```python
from build123d import *

# Parameters (mm, degrees)
SKETCH1_W                        = 40.9
SKETCH1_H                        = 40.9
BOSS_EXTRUDE1_DEPTH              = 40
CUT_EXTRUDE1_START               = -30.475
SKETCH3_W                        = 28.2
SKETCH3_H                        = 28.2
CUT_EXTRUDE1_DEPTH               = 30.475
FILLET1_R                        = 9.525
CIRPATTERN1_COUNT                = 2
CIRPATTERN1_ANGLE                = 90
SKETCH6_W                        = 2.5527
SKETCH6_H                        = 9.525
F_1_4_20_TAPPED_HOLE1_AT_2_COUNT = 2
F_1_4_20_TAPPED_HOLE1_AT_2_PITCH = 19.05
F_1_4_20_TAPPED_HOLE1_AT_3_COUNT = 2
F_1_4_20_TAPPED_HOLE1_AT_3_PITCH = 26.940768363
F_1_4_20_TAPPED_HOLE1_AT_4_COUNT = 2
F_1_4_20_TAPPED_HOLE1_AT_4_PITCH = 19.05


with BuildPart() as part:
    # Sketch1 → Boss-Extrude1 (new body)
    with BuildSketch(Plane(origin=(0, 0, 0), x_dir=(1, 0, 0), z_dir=(0, 1, 0))):
        Rectangle(SKETCH1_W, SKETCH1_H)
    extrude(amount=BOSS_EXTRUDE1_DEPTH)

    # Sketch3 → Cut-Extrude1 (cut)
    with BuildSketch(Plane(origin=(0, 40, 0), x_dir=(1, 0, 0), z_dir=(0, 1, 0)).offset(CUT_EXTRUDE1_START)):
        Rectangle(SKETCH3_W, SKETCH3_H)
    extrude(amount=CUT_EXTRUDE1_DEPTH, mode=Mode.SUBTRACT)

    # Fillet1
    fillet1_edges = [part.edges().sort_by_distance(p)[0] for p in [
        (14.1, 24.7625, 14.1),
        (14.1, 24.7625, -14.1),
        (-14.1, 24.7625, -14.1),
        (-14.1, 24.7625, 14.1),
    ]]
    fillet(fillet1_edges, radius=FILLET1_R)

    # Sketch4 → 5/16-18 Tapped Hole1 (revolve, cut)
    with BuildSketch(Plane(origin=(0, 25, 20.45), x_dir=(0, -1, 0), z_dir=(1, 0, 0))):
        Polygon((0, 0), (0, 24.884648974), (3.2639, 22.9235), (3.2639, 0), align=None)
    f_5_16_18_tapped_hole1 = revolve(axis=Axis((0, 25, 26.8), (0, 0, -1)), mode=Mode.SUBTRACT)

    # CirPattern1: 5/16-18 Tapped Hole1 ×2 about axis
    cirpattern1_axis = Axis((0, -2, 0), (0, -1, 0))
    for i in range(1, CIRPATTERN1_COUNT):
        add(f_5_16_18_tapped_hole1.rotate(cirpattern1_axis, i * CIRPATTERN1_ANGLE / (CIRPATTERN1_COUNT - 1)), mode=Mode.SUBTRACT)

    # Sketch6 → 1/4-20 Tapped Hole1 (revolve, cut)
    with BuildSketch(Plane(origin=(-9.525, 9.525, -9.525), x_dir=(0, 0, 1), z_dir=(1, 0, 0))):
        with Locations((1.27635, 4.7625)):
            Rectangle(SKETCH6_W, SKETCH6_H)
    f_1_4_20_tapped_hole1 = revolve(axis=Axis((-9.525, 15.875, -9.525), (0, -1, 0)), mode=Mode.SUBTRACT)

    # 1/4-20 Tapped Hole1 at 2: 1/4-20 Tapped Hole1 ×2
    with Locations(*[(i * F_1_4_20_TAPPED_HOLE1_AT_2_PITCH, 0, 0) for i in range(1, F_1_4_20_TAPPED_HOLE1_AT_2_COUNT)]):
        add(f_1_4_20_tapped_hole1, mode=Mode.SUBTRACT)

    # 1/4-20 Tapped Hole1 at 3: 1/4-20 Tapped Hole1 ×2
    with Locations(*[Vector(0.7071067811865476, 0, 0.7071067811865475) * (i * F_1_4_20_TAPPED_HOLE1_AT_3_PITCH) for i in range(1, F_1_4_20_TAPPED_HOLE1_AT_3_COUNT)]):
        add(f_1_4_20_tapped_hole1, mode=Mode.SUBTRACT)

    # 1/4-20 Tapped Hole1 at 4: 1/4-20 Tapped Hole1 ×2
    with Locations(*[(0, 0, i * F_1_4_20_TAPPED_HOLE1_AT_4_PITCH) for i in range(1, F_1_4_20_TAPPED_HOLE1_AT_4_COUNT)]):
        add(f_1_4_20_tapped_hole1, mode=Mode.SUBTRACT)


solid = part.part
```
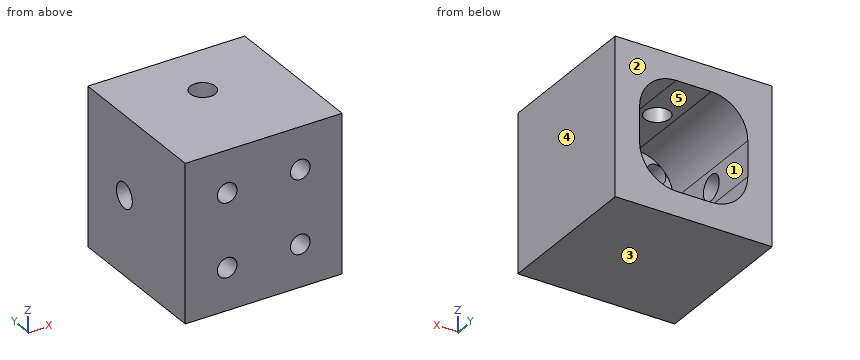
Geometry check sheet. Reference: the model listing, model coordinates, mm. Face numbers are marked on the shaded views. A direction names the side the tool comes from. Round coordinates to 2 decimals unless told otherwise and drop trailing zeros. Loops run counter-clockwise (first coordinate to the right, second up) from the corner with the lowest first, then second, coordinate; pieces in that order, holes last. Notation, with made-up numbers: M 80,38 L 131,38 A30 ccw 131,68 Z; hole C -24.75,32.25 d10. An arc over 180 degrees is marked long. Return JSON: item names as keys, results as strings. Group by question number.
(1) Section check B-B, the plane y = 25. Enter the section's corners in (x, z) (3 decimals), and give its area (3 significant figures).
(2) Mould release check, pull along Z, two halves, no side actions. Record for the marked faces 3, 4 and 5: pulls with the +Z half, pulls with the -Z half, needs draft (parallel to the pull), parting line crosses it, or undercut.
(3) Scan lines: line 1 along X through (y, z) = (25, 17.25); line 2 along X through (y, z) = (25, -11); line 3 along Z through (x, y) = (8.5, 8). Record each from-to range of solid material in increasing order. Write a range as [from, to].
(4) Section check C-C, the plane z = 0. Enter the section's corners in (x, y) (3 decimals), and give its area (3 significant figures).
(5) Section check D-D, the plane y = 31. Enter the section's corners in (x, z) (3 decimals), and give its area (3 significant figures).
(6) Set-up check for the marked faces 1 and 2: record each of +Z, -Z, +X, -X, +Y, -Y from which the full face is reachable in a straight line by a thin tool's end or side.
(7) Section check A-A, the plane x = 0. Enter the section's corners in (y, z) (3 decimals), and give its area (3 significant figures).
Data:
{
 "1": {"outline": "M -20.45,-20.45 L 20.45,-20.45 L 20.45,20.45 L 3.264,20.45 L 3.264,14.1 L 4.575,14.1 A9.525 cw 14.1,4.575 L 14.1,-4.575 A9.525 cw 4.575,-14.1 L -4.575,-14.1 A9.525 cw -14.1,-4.575 L -14.1,-3.264 L -20.45,-3.264 Z; M -20.45,3.264 L -14.1,3.264 L -14.1,4.575 A9.525 cw -4.575,14.1 L -3.264,14.1 L -3.264,20.45 L -20.45,20.45 Z", "area": "873 mm²"},
 "2": {"face 3": "pulls with the -Z half", "face 4": "needs draft", "face 5": "undercut"},
 "3": {"line 1": "[-20.45, -3.26], [3.26, 20.45]", "line 2": "[-20.45, -11.61], [11.61, 20.45]", "line 3": "[-20.45, -11.86], [-7.19, 7.19], [11.86, 20.45]"},
 "4": {"outline": "M -20.45,0 L 20.45,0 L 20.45,40 L 14.1,40 L 14.1,9.525 L -14.1,9.525 L -14.1,21.736 L -20.45,21.736 Z; M -20.45,28.264 L -14.1,28.264 L -14.1,40 L -20.45,40 Z", "area": "735 mm²"},
 "5": {"outline": "M -20.45,-20.45 L 20.45,-20.45 L 20.45,20.45 L -20.45,20.45 Z; hole M -14.1,-4.575 A9.525 ccw -4.575,-14.1 L 4.575,-14.1 A9.525 ccw 14.1,-4.575 L 14.1,4.575 A9.525 ccw 4.575,14.1 L -4.575,14.1 A9.525 ccw -14.1,4.575 Z", "area": "955 mm²"},
 "6": {"face 1": "+Y", "face 2": "+Z, -Z, +X, -X, +Y"},
 "7": {"outline": "M 0,-20.45 L 40,-20.45 L 40,-14.1 L 9.525,-14.1 L 9.525,14.1 L 21.736,14.1 L 21.736,20.45 L 0,20.45 Z; M 28.264,14.1 L 40,14.1 L 40,20.45 L 28.264,20.45 Z", "area": "735 mm²"}
}
